```python
from build123d import *

# Parameters (mm, degrees)
SKETCH_1_W      = 107.764696886
SKETCH_1_H      = 59.957319102
EXTRUDE_1_DEPTH = 33
FILLET_1_R      = 10
FILLET_2_R      = 10
FILLET_4_R      = 10
FILLET_5_R      = 10
SKETCH_2_R      = 2.546868178
EXTRUDE_2_DEPTH = 3


with BuildPart() as part:
    # 草图1 → 凸台-拉伸1 (new body)
    with BuildSketch(Plane.XY):
        Rectangle(SKETCH_1_W, SKETCH_1_H)
    extrude(amount=EXTRUDE_1_DEPTH)

    # 圆角1
    fillet_1_edges = [part.edges().sort_by_distance(p)[0] for p in [
        (53.882348443, 29.978659551, 16.5),
    ]]
    fillet(fillet_1_edges, radius=FILLET_1_R)

    # 圆角2
    fillet_2_edges = [part.edges().sort_by_distance(p)[0] for p in [
        (53.882348443, -29.978659551, 16.5),
    ]]
    fillet(fillet_2_edges, radius=FILLET_2_R)

    # 圆角4
    fillet_4_edges = [part.edges().sort_by_distance(p)[0] for p in [
        (-53.882348443, 29.978659551, 16.5),
    ]]
    fillet(fillet_4_edges, radius=FILLET_4_R)

    # 圆角5
    fillet_5_edges = [part.edges().sort_by_distance(p)[0] for p in [
        (-53.882348443, -29.978659551, 16.5),
    ]]
    fillet(fillet_5_edges, radius=FILLET_5_R)

    # 草图2 → 凸台-拉伸2 (add)
    with BuildSketch(Plane(origin=(0, 0, 0), x_dir=(-1, 0, 0), z_dir=(0, 0, -1))):
        with Locations(Location((-36.108931064, 0, 0), (0, 0, 180))):
            Circle(SKETCH_2_R)
    extrude(amount=EXTRUDE_2_DEPTH)


solid = part.part
```
Geometry: final body of the model. Coordinates: model frame, mm. A direction names the side the tool comes from. Coordinates: 2 decimals unless noted, no trailing zeros. Loops run counter-clockwise (first coordinate to the right, second up) from the corner with the lowest first, then second, coordinate; pieces in that order, holes last. Notation, with made-up numbers: M 30,53 L 51,53 A32 ccw 51,79 Z; hole C 73,79 d9. An arc over 180 degrees is marked long. Put each result on its own line as item: value.
(1) Cut plane A-A on y = 0. Return the cut outline in (x, z), then the cut area to 3 significant figures.
Answer sheet:
outline: M -53.88,0 L 33.56,0 L 33.56,-3 L 38.66,-3 L 38.66,0 L 53.88,0 L 53.88,33 L -53.88,33 Z
area: 3,570 mm^2
(2) Cut plane C-C on y = 11. Return the cut outline in (x, z).
Answer sheet:
outline: M -53.88,0 L 53.88,0 L 53.88,33 L -53.88,33 Z
(3) First-contact query: pin 1 (4 mm diameter, centred on x = -28, y = 10.5, fed in from -Z). Flat tip, straight axial feed; report the tip coordinate or a pass-through.
Answer sheet:
pin 1: stops at z = 0
(4) Material intervals for probe 1 along Z at (x, y) = (10, 8); probe 2 along Y at (x, z) = (-44, 27.5); probe 3 along X at (y, z) = (22, 25.5), sorted ascending.
Answer sheet:
probe 1: z = 0 to 33
probe 2: y = -29.98 to 29.98
probe 3: x = -53.68 to 53.68
(5) Access query for faces 1 (the face through (38.538, -0.765, -1.479)), 2 (the face through (-1, 29.979, 16)). Directions: +Z, -Z, +X, -X, +Y, -Y. A direction counts if a zero-diameter tool reaches every point of the face in a straight line with its end or side. Return the directions, or none.
Answer sheet:
face 1: -Z
face 2: +Z, -Z, +X, -X, +Y
(6) Cut plane B-B on x = 25.5. Return the cut outline in (y, z).
Answer sheet:
outline: M -29.98,0 L 29.98,0 L 29.98,33 L -29.98,33 Z
